Autodesk Inventor part; units mm, degrees
ref_plane "YZ Plane" through (0, 0, 0) normal (1, 0, 0) x (0, 1, 0)
ref_plane "XZ Plane" through (0, 0, 0) normal (0, 1, 0) x (-1, 0, 0)
ref_plane "XY Plane" through (0, 0, 0) normal (0, 0, 1) x (1, 0, 0)
sketch "Sketch1" plane through (0, 0, 0) normal (0, 0, 1) x (1, 0, 0)
  line L0 (-2.55, -10) -> (-2.55, -9.25)
  line L1 (-2.55, -9.25) -> (-2.05, -9.25)
  line L2 (-7.75, -10) -> (-2.55, -10)
  line L3 (-2.05, -9.25) -> (-2.05, -7)
  line L4 (-2.05, -7) -> (-3.05, -7)
  line L5 (-3.05, -9.1) -> (-3.05, -7)
  line L6 (-3.05, -9.1) -> (-5.125, -9.1)
  line L7 (-5.125, -9.1) -> (-5.125, -5.8321)
  line L8 (-8, -9.25) -> (-5.775, -9.25)
  line L9 (-5.775, -9.25) -> (-5.775, -5.775)
  line L10 (-2.2929, -3) -> (2.2929, -3)
  line L11 (3, -2.2929) -> (3, 2.2929)
  line L12 (2.2929, 3) -> (-2.2929, 3)
  line L13 (-3, 2.2929) -> (-3, -2.2929)
  line L14 (-2.2929, -3) -> (-5.125, -5.8321)
  line L15 (-3, -2.2929) -> (-5.8321, -5.125)
  line L16 (-9.1, -5.125) -> (-5.8321, -5.125)
  line L17 (-9.25, -5.775) -> (-5.775, -5.775)
  line L18 (-9.25, -8) -> (-9.25, -5.775)
  line L19 (-10, -7.75) -> (-10, -2.55)
  line L20 (-9.1, -3.05) -> (-9.1, -5.125)
  line L21 (-9.1, -3.05) -> (-7, -3.05)
  line L22 (-9.25, -2.55) -> (-9.25, -2.05)
  line L23 (-9.25, -2.05) -> (-7, -2.05)
  line L24 (-7, -2.05) -> (-7, -3.05)
  line L25 (-10, -2.55) -> (-9.25, -2.55)
  arc A0 (-9.25, -8) -> (-8, -9.25) centre (-8, -8) ccw
  arc A1 (-10, -7.75) -> (-7.75, -10) centre (-7.75, -7.75) ccw
  line L26 (3, -2.2929) -> (5.8321, -5.125)
  line L27 (2.2929, -3) -> (5.125, -5.8321)
  line L28 (5.775, -9.25) -> (5.775, -5.775)
  line L29 (8, -9.25) -> (5.775, -9.25)
  line L30 (7.75, -10) -> (2.55, -10)
  line L31 (3.05, -9.1) -> (5.125, -9.1)
  line L32 (2.55, -10) -> (2.55, -9.25)
  line L33 (3.05, -9.1) -> (3.05, -7)
  line L34 (2.05, -9.25) -> (2.05, -7)
  line L35 (2.55, -9.25) -> (2.05, -9.25)
  line L36 (2.05, -7) -> (3.05, -7)
  line L37 (5.125, -9.1) -> (5.125, -5.8321)
  arc A2 (8, -9.25) -> (9.25, -8) centre (8, -8) ccw
  arc A3 (7.75, -10) -> (10, -7.75) centre (7.75, -7.75) ccw
  line L38 (9.25, -8) -> (9.25, -5.775)
  line L39 (10, -7.75) -> (10, -2.55)
  line L40 (9.25, -5.775) -> (5.775, -5.775)
  line L41 (9.1, -5.125) -> (5.8321, -5.125)
  line L42 (9.1, -3.05) -> (7, -3.05)
  line L43 (7, -2.05) -> (7, -3.05)
  line L44 (9.25, -2.05) -> (7, -2.05)
  line L45 (9.25, -2.55) -> (9.25, -2.05)
  line L46 (10, -2.55) -> (9.25, -2.55)
  line L47 (9.1, -3.05) -> (9.1, -5.125)
  line L48 (2.2929, 3) -> (5.125, 5.8321)
  line L49 (3, 2.2929) -> (5.8321, 5.125)
  line L50 (9.25, 5.775) -> (5.775, 5.775)
  line L51 (9.25, 8) -> (9.25, 5.775)
  line L52 (10, 7.75) -> (10, 2.55)
  line L53 (9.1, 3.05) -> (9.1, 5.125)
  line L54 (10, 2.55) -> (9.25, 2.55)
  line L55 (9.1, 3.05) -> (7, 3.05)
  line L56 (9.25, 2.05) -> (7, 2.05)
  line L57 (9.25, 2.55) -> (9.25, 2.05)
  line L58 (7, 2.05) -> (7, 3.05)
  line L59 (9.1, 5.125) -> (5.8321, 5.125)
  arc A4 (9.25, 8) -> (8, 9.25) centre (8, 8) ccw
  arc A5 (10, 7.75) -> (7.75, 10) centre (7.75, 7.75) ccw
  line L60 (8, 9.25) -> (5.775, 9.25)
  line L61 (7.75, 10) -> (2.55, 10)
  line L62 (5.775, 9.25) -> (5.775, 5.775)
  line L63 (5.125, 9.1) -> (5.125, 5.8321)
  line L64 (3.05, 9.1) -> (3.05, 7)
  line L65 (2.05, 7) -> (3.05, 7)
  line L66 (2.05, 9.25) -> (2.05, 7)
  line L67 (2.55, 9.25) -> (2.05, 9.25)
  line L68 (2.55, 10) -> (2.55, 9.25)
  line L69 (3.05, 9.1) -> (5.125, 9.1)
  line L70 (-3, 2.2929) -> (-5.8321, 5.125)
  line L71 (-2.2929, 3) -> (-5.125, 5.8321)
  line L72 (-5.775, 9.25) -> (-5.775, 5.775)
  line L73 (-8, 9.25) -> (-5.775, 9.25)
  line L74 (-7.75, 10) -> (-2.55, 10)
  line L75 (-3.05, 9.1) -> (-5.125, 9.1)
  line L76 (-2.55, 10) -> (-2.55, 9.25)
  line L77 (-3.05, 9.1) -> (-3.05, 7)
  line L78 (-2.05, 9.25) -> (-2.05, 7)
  line L79 (-2.55, 9.25) -> (-2.05, 9.25)
  line L80 (-2.05, 7) -> (-3.05, 7)
  line L81 (-5.125, 9.1) -> (-5.125, 5.8321)
  arc A6 (-8, 9.25) -> (-9.25, 8) centre (-8, 8) ccw
  arc A7 (-7.75, 10) -> (-10, 7.75) centre (-7.75, 7.75) ccw
  line L82 (-9.25, 8) -> (-9.25, 5.775)
  line L83 (-10, 7.75) -> (-10, 2.55)
  line L84 (-9.25, 5.775) -> (-5.775, 5.775)
  line L85 (-9.1, 5.125) -> (-5.8321, 5.125)
  line L86 (-9.1, 3.05) -> (-7, 3.05)
  line L87 (-7, 2.05) -> (-7, 3.05)
  line L88 (-9.25, 2.05) -> (-7, 2.05)
  line L89 (-9.25, 2.55) -> (-9.25, 2.05)
  line L90 (-10, 2.55) -> (-9.25, 2.55)
  line L91 (-9.1, 3.05) -> (-9.1, 5.125)
  circle A8 centre (0, 0) radius 2
  point P0 (-10, -10)
  point P1 (10, -10)
  point P2 (10, 10)
  point P3 (-10, 10)
  dimension "d2" = 0.75
  dimension "d3" = 7.45
  dimension "d4" = 2.25
  dimension "d5" = 1
  dimension "d6" = 2.1
  dimension "d7" = 0.75
  dimension "d8" = 0.65
  dimension "d9" = 1.25
  dimension "d10" = 2.25
  dimension "d11" = 360
  dimension "d12" = 4
  dimension "d13" = 20
extrude "Extrusion1" add sketch "Sketch1" along normal blind 300
properties part number "2020 dai 300"
Geometry: final body of the model. Coordinates: model frame, mm. Round coordinates to 2 decimals unless told otherwise and drop trailing zeros. Write each question's results on one line, items separated by ' | '. Start each with the question number.
1) Line query: probe 1 along Y at (x, z) = (2.25, 262); probe 2 along Y at (x, z) = (0, 184.5); probe 3 along Y at (x, z) = (-4.5, 286). Output: solid intervals per line, ascending. Write a range as [from, to].
2) First-contact query: P1, Ø0.6, axis at y = -9.5, z = 157.5, coming from the +X side; P2, Ø0.6, axis at x = -9.5, z = 154, coming from the +Y side; P3, Ø1, axis at x = -7.5, y = 0.5, coming from the -Z side; P4, Ø0.8, axis at y = -9.5, z = 207.5, coming from the -X side. Flat tips, straight axial feed; report the tip coordinate or a pass-through.
3) Cut plane A-A on z = 92.5. Count the separate pieces of the cut face and the enclosed holes in it, then the cut area to 3 significant figures.
4) Mould query, pull axis Y, two halves, no side actions, for faces 1 (the face through (10, -5, 148)), 2 (the face through (3, 0, 148)), 3 (the face through (-3, 0, 148)), 4 (the face through (-5, -10, 148)). Classes: released by +Y, released by -Y, zero draft, split by the parting line, or undercut.
Verdict:
1) probe 1: y = [-9.25, -7], [-3, 3], [7, 9.25] | probe 2: y = [-3, -2], [2, 3] | probe 3: y = [-10, -9.1], [-5.21, -3.79], [3.79, 5.21], [9.1, 10]
2) P1: stops at x = 9.47 | P2: stops at y = 9.47 | P3: passes through | P4: stops at x = -9.55
3) separate pieces: 1 | enclosed holes: 5 | area: 117 mm2
4) face 1: zero draft | face 2: undercut | face 3: undercut | face 4: released by -Y
